from build123d import *

# Parameters (mm, degrees)
SKETCH1_R           = 5
BOSS_EXTRUDE1_DEPTH = 60
BOSS_EXTRUDE2_START = -43
SKETCH2_R           = 5.5
BOSS_EXTRUDE2_DEPTH = 3
CHAMFER1_SIZE       = 1
BOSS_EXTRUDE3_START = -7
SKETCH3_R           = 5.5
BOSS_EXTRUDE3_DEPTH = 3


with BuildPart() as part:
    # Sketch1 → Boss-Extrude1 (new body)
    with BuildSketch(Plane(origin=(0, 0, 0), x_dir=(1, 0, 0), z_dir=(0, 1, 0))):
        with Locations(Location((0, 0, 0), (0, 0, 270))):
            Circle(SKETCH1_R)
    extrude(amount=BOSS_EXTRUDE1_DEPTH)

    # Sketch2 → Boss-Extrude2 (add)
    with BuildSketch(Plane(origin=(0, 60, 0), x_dir=(1, 0, 0), z_dir=(0, 1, 0)).offset(BOSS_EXTRUDE2_START)):
        with Locations(Location((0, 0, 0), (0, 0, 270))):
            Circle(SKETCH2_R)
    extrude(amount=BOSS_EXTRUDE2_DEPTH)

    # Chamfer1
    chamfer1_edges = [part.edges().sort_by_distance(p)[0] for p in [
        (0, 0, -5),
    ]]
    chamfer(chamfer1_edges, length=CHAMFER1_SIZE)

    # Sketch3 → Boss-Extrude3 (add)
    with BuildSketch(Plane.XZ.offset(BOSS_EXTRUDE3_START)):
        with Locations(Location((0, 0, 0), (0, 0, 90))):
            Circle(SKETCH3_R)
    extrude(amount=-BOSS_EXTRUDE3_DEPTH)


solid = part.part
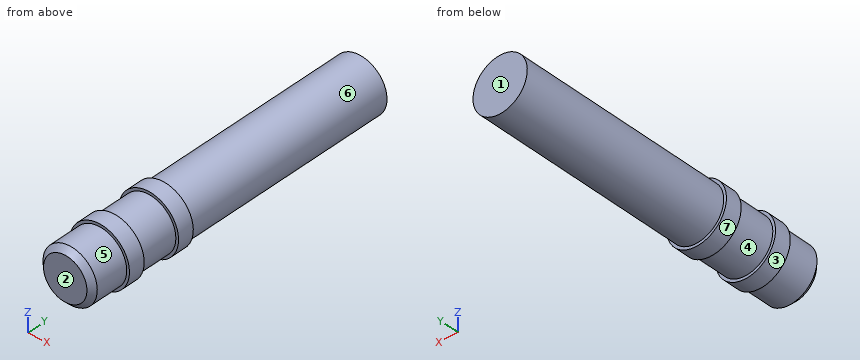
Model file for the job. Use its own axes, mm. Face numbers are marked on the shaded views. A direction names the side the tool comes from. Coordinates: 2 decimals unless noted, no trailing zeros. Loops run counter-clockwise (first coordinate to the right, second up) from the corner with the lowest first, then second, coordinate; pieces in that order, holes last. Notation, with made-up numbers: (-36.75, 9.5) -> (-32.75, 9.5) arc R13 cw to (-32.75, 27.5) -> close; hole circle Ø2 at (-25.5, 26.25). An arc over 180 degrees is marked (long way). Use one line per item in the form item = value. Start each with the question number.
(1) Tool access for the marked faces 5, 6 and 7: list every direction of +Z, -Z, +X, -X, +Y, -Y with a clear straight run to the whole face (end or side of a thin tool).
(2) Probe probe 1 along X at (y, z) = (55, -0.25); probe 2 along Y at (x, z) = (-3.25, 4.25); probe 3 along X at (y, z) = (26, -3). List the from-to ranges inside material, lowest first. Write a range as from..to.
(3) Cut at A-A on z = 0. Give the cut face in (x, y).
(4) Cut at B-B on x = 0. Give the cut face in (y, z).
(5) Pull direction Y, two halves, no side cores. Call the marked faces 1, 2, 3 and 4: pulls with the +Y half, pulls with the -Y half, needs draft (parallel to the pull), parting line crosses it, or undercut.
(6) Cut at C-C on y = 9. Give the cut face in (x, z).
(7) Flat gauge pins, fed straight in: pin 1 (3 mm diameter, centred on x = 3, y = 23.5, fed in from +Z); pin 2 (1.5 mm diameter, centred on x = -4, y = 46.5, fed in from +Z); pin 3 (4 mm diameter, centred on x = 1, y = 34, fed in from -Z). Where does each tip first touch, or does it go through?
(8) Cut at D-D on y = 28.5. Give the cut face in (x, z).
Values:
q1.face_5 = -Y
q1.face_6 = +Y
q1.face_7 = +Y, -Y
q2.probe_1 = -4.99..4.99
q2.probe_2 = 7..10, 17..20
q2.probe_3 = -4..4
q3.outline = (-5.5, 7) -> (-5, 7) -> (-5, 1) -> (-4, 0) -> (4, 0) -> (5, 1) -> (5, 7) -> (5.5, 7) -> (5.5, 10) -> (5, 10) -> (5, 17) -> (5.5, 17) -> (5.5, 20) -> (5, 20) -> (5, 60) -> (-5, 60) -> (-5, 20) -> (-5.5, 20) -> (-5.5, 17) -> (-5, 17) -> (-5, 10) -> (-5.5, 10) -> close
q4.outline = (0, -4) -> (1, -5) -> (7, -5) -> (7, -5.5) -> (10, -5.5) -> (10, -5) -> (17, -5) -> (17, -5.5) -> (20, -5.5) -> (20, -5) -> (60, -5) -> (60, 5) -> (20, 5) -> (20, 5.5) -> (17, 5.5) -> (17, 5) -> (10, 5) -> (10, 5.5) -> (7, 5.5) -> (7, 5) -> (1, 5) -> (0, 4) -> close
q5.face_1 = pulls with the +Y half
q5.face_2 = pulls with the -Y half
q5.face_3 = needs draft
q5.face_4 = undercut
q6.outline = circle Ø11 at (0, 0)
q7.pin_1 = 4.77
q7.pin_2 = 3.8
q7.pin_3 = -5
q8.outline = circle Ø10 at (0, 0)
